```python
from build123d import *

# Parameters (mm, degrees)
SKETCH_3_W      = 34
SKETCH_3_H      = 16
EXTRUDE_3_DEPTH = 3
FILLET_1_R      = 1


with BuildPart() as part:
    # 草图3 → 凸台-拉伸3 (new body)
    with BuildSketch(Plane(origin=(0, 0, 0), x_dir=(1, 0, 0), z_dir=(0, 1, 0))):
        Rectangle(SKETCH_3_W, SKETCH_3_H)
        with BuildLine():
            ThreePointArc((-13.1, -4.35), (-11.85, -3.1), (-13.1, -1.85))
            ThreePointArc((-13.1, -1.85), (-14.35, -3.1), (-13.1, -4.35))
        make_face(mode=Mode.SUBTRACT)
        with BuildLine():
            ThreePointArc((13.1, -4.35), (14.35, -3.1), (13.1, -1.85))
            ThreePointArc((13.1, -1.85), (11.85, -3.1), (13.1, -4.35))
        make_face(mode=Mode.SUBTRACT)
        with BuildLine():
            ThreePointArc((13.1, 4.35), (11.85, 3.100000001), (13.1, 1.850000001))
            ThreePointArc((13.1, 1.850000001), (14.349999999, 3.1), (13.1, 4.35))
        make_face(mode=Mode.SUBTRACT)
        with BuildLine():
            ThreePointArc((-13.1, 1.85), (-11.85, 3.1), (-13.1, 4.349999999))
            ThreePointArc((-13.1, 4.349999999), (-14.35, 3.1), (-13.1, 1.85))
        make_face(mode=Mode.SUBTRACT)
    extrude(amount=EXTRUDE_3_DEPTH)

    # 圆角1
    fillet_1_edges = [part.edges().sort_by_distance(p)[0] for p in [
        (-17, 1.5, -8),
        (17, 1.5, -8),
        (17, 1.5, 8),
        (-17, 1.5, 8),
    ]]
    fillet(fillet_1_edges, radius=FILLET_1_R)


solid = part.part
```
The model under review builds one solid part; all positions refer to its coordinate system, in mm. Round coordinates to 2 decimals unless told otherwise and drop trailing zeros. Order: outer loops, then holes, each group sorted by start corner. A loop starts at its lowest first (then second) coordinate and runs counter-clockwise, first axis right, second up. Notation, with made-up numbers: (41.25, -29.75) - (54.25, -29.75) arc R13 cw to (54.25, -16.75) - close; hole circle Ø8 at (2, 2.25). An arc over 180 degrees is marked (long way). Answer in a Markdown table with one row per item.
(1) Mouldability with a two-part tool opening along X and no side actions: class faces 1 (the face through (-11.991, 1.479, 2.523)), 2 (the face through (16.699, 1.521, -7.715)), 3 (the face through (-16.715, 1.521, 7.699)) as released by +X, released by -X, zero draft, split by the parting line, or undercut.
Result set:
| item | result |
|---|---|
| face 1 | undercut |
| face 2 | released by +X |
| face 3 | released by -X |
(2) Take a section at C-C on y = 1.5. Write out the cut boundary in (x, z), plus the area to 3 significant figures.
Result set:
| item | result |
|---|---|
| outline | (-17, -7) arc R1 ccw to (-16, -8) - (16, -8) arc R1 ccw to (17, -7) - (17, 7) arc R1 ccw to (16, 8) - (-16, 8) arc R1 ccw to (-17, 7) - close; hole circle Ø2.5 at (-13.1, -3.1); hole circle Ø2.5 at (-13.1, 3.1); hole circle Ø2.5 at (13.1, -3.1); hole circle Ø2.5 at (13.1, 3.1) |
| area | 524 mm2 |
(3) Clearance check with a flat-ended pin moving along its axis: P1, Ø6, axis at x = -12, z = 2, coming from the -Y side. State where the tip first meets the part, or that it passes through.
Result set:
| item | result |
|---|---|
| P1 | stops at y = 0 |
(4) Take a section at B-B on z = 3.1. Write out the cut boundary in (x, y), plus the area to 3 significant figures.
Result set:
| item | result |
|---|---|
| outline | (-17, 0) - (-14.35, 0) - (-14.35, 3) - (-17, 3) - close; (-11.85, 0) - (11.85, 0) - (11.85, 3) - (-11.85, 3) - close; (14.35, 0) - (17, 0) - (17, 3) - (14.35, 3) - close |
| area | 87.0 mm2 |
(5) Take a section at A-A on x = 13.1. Write out the cut boundary in (y, z).
Result set:
| item | result |
|---|---|
| outline | (0, -8) - (3, -8) - (3, -4.35) - (0, -4.35) - close; (0, -1.85) - (3, -1.85) - (3, 1.85) - (0, 1.85) - close; (0, 4.35) - (3, 4.35) - (3, 8) - (0, 8) - close |
(6) For line 1 (Z direction, x = -13.1, y = 2.1); line 2 (X direction, y = 2.35, z = 3.1); line 3 (Z direction, x = -14, y = 1.65), list the stretches that pass through material, from the lowest coordinate up. Write a range as from..to.
Result set:
| item | result |
|---|---|
| line 1 | z = -8..-4.35, -1.85..1.85, 4.35..8 |
| line 2 | x = -17..-14.35, -11.85..11.85, 14.35..17 |
| line 3 | z = -8..-3.97, -2.23..2.23, 3.97..8 |
